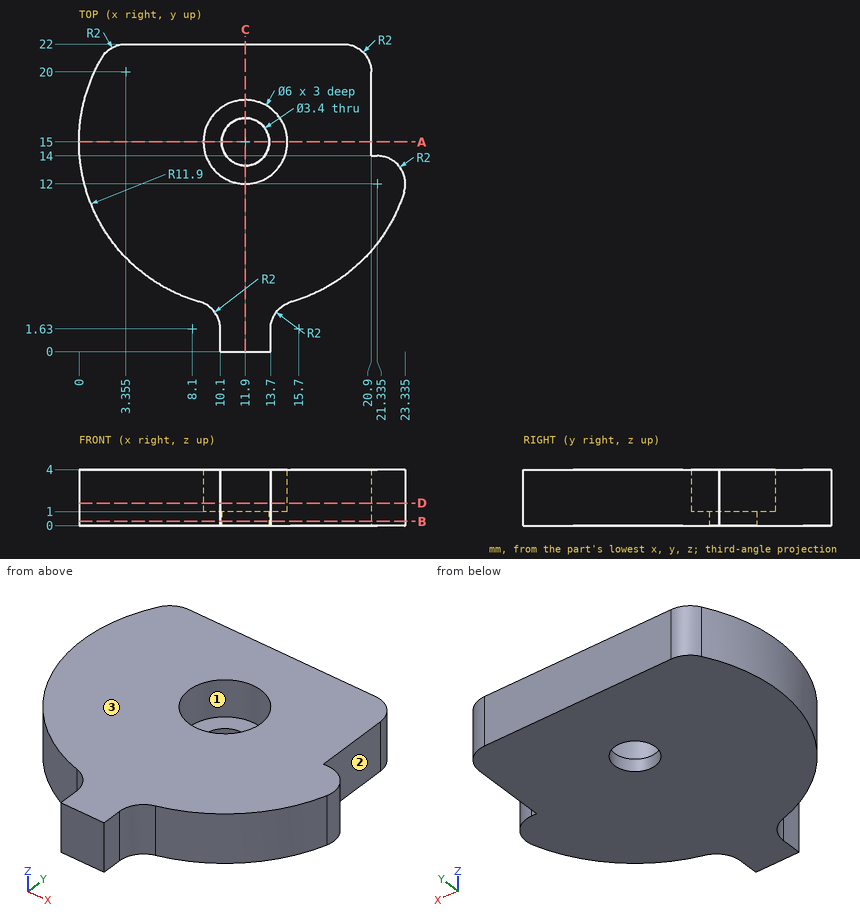
Input: dimensioned drawing with shaded views. Units: mm. Origin: part minimum x, y, z. Coordinates: 2 decimals unless noted, no trailing zeros. Write each loop counter-clockwise with the first axis right and the second up, starting at its lowest first coordinate (ties: lowest second). Pieces come first, ordered by that corner, then holes. Notation, with made-up numbers: (67, 43.5) -> (105, 43.5) arc R22 ccw to (105, 58.5) -> close; hole circle Ø11 at (73, 30). An arc over 180 degrees is marked (long way). Return JSON: item names as keys, results as strings. Group by question number.
1) Mould query, pull axis X, two halves, no side actions, for the marked faces 1, 2 and 3. Classes: +X half, -X half, draft (parallel to the pull), parting line (faces both ways), or undercut.
2) Section query A-A, the plane y = 15. Return loops of the section in (x, z).
3) Ray query, line 1 along X through (y, z) = (15, 0.3); line 2 along Y through (x, z) = (11.9, 0.8); line 3 along Y through (x, z) = (11.9, 3.3). Return the intervals inside material, ascending.
4) Section query C-C, the plane x = 11.9. Return loops of the section in (y, z).
5) Section query D-D, the plane z = 1.6. Return loops of the section in (x, y) (1 decimal), plus the area to 3 significant figures.
6) Contact query for flat-ended pins moving along their axis: P1, Ø1, axis at y = 13.5, z = 2.5, coming from the +X side; P2, Ø1.3, axis at y = 1, z = 1.5, coming from the +X side; P3, Ø1.5, axis at x = 5.5, z = 2.5, coming from the -Y side; P4, Ø2.5, axis at x = 11.9, y = 15, coming from the +Z side. Output: stop coordinate, or through.
7) Section query B-B, the plane z = 0.3. Return loops of the section in (x, y) (1 decimal).
From the geometry:
{
 "1": {"face 1": "undercut", "face 2": "+X half", "face 3": "draft"},
 "2": {"outline": "(0, 0) -> (10.2, 0) -> (10.2, 1) -> (8.9, 1) -> (8.9, 4) -> (0, 4) -> close; (13.6, 0) -> (20.9, 0) -> (20.9, 4) -> (14.9, 4) -> (14.9, 1) -> (13.6, 1) -> close"},
 "3": {"line 1": "0 to 10.2, 13.6 to 20.9", "line 2": "0 to 13.3, 16.7 to 22", "line 3": "0 to 12, 18 to 22"},
 "4": {"outline": "(0, 0) -> (13.3, 0) -> (13.3, 1) -> (12, 1) -> (12, 4) -> (0, 4) -> close; (16.7, 0) -> (22, 0) -> (22, 4) -> (18, 4) -> (18, 1) -> (16.7, 1) -> close"},
 "5": {"outline": "(1.6, 21) arc R11.9 ccw to (8.6, 3.6) arc R2 cw to (10.1, 1.6) -> (10.1, 0) -> (13.7, 0) -> (13.7, 1.6) arc R2 cw to (15.2, 3.6) arc R11.9 ccw to (23.2, 11.4) arc R2 ccw to (21.3, 14) -> (20.9, 14) -> (20.9, 20) arc R2 ccw to (18.9, 22) -> (3.4, 22) arc R2 ccw to start; hole circle Ø6 at (11.9, 15)", "area": "342 mm²"},
 "6": {"P1": "x = 23.07", "P2": "x = 13.7", "P3": "y = 4.53", "P4": "through"},
 "7": {"outline": "(1.6, 21) arc R11.9 ccw to (8.6, 3.6) arc R2 cw to (10.1, 1.6) -> (10.1, 0) -> (13.7, 0) -> (13.7, 1.6) arc R2 cw to (15.2, 3.6) arc R11.9 ccw to (23.2, 11.4) arc R2 ccw to (21.3, 14) -> (20.9, 14) -> (20.9, 20) arc R2 ccw to (18.9, 22) -> (3.4, 22) arc R2 ccw to start; hole circle Ø3.4 at (11.9, 15)"}
}
